```python
from build123d import *

# Parameters (mm, degrees)
SKETCH2_W               = 152.4
SKETCH2_H               = 44.45
BASE_FLANGE1_DEPTH      = 6.07314
CUT_EXTRUDE1_DEPTH      = 159.86612455
CUT_EXTRUDE1_DEPTH_BACK = 159.86612455


# Sheet-metal steps are written as plain solids
with BuildPart() as part:
    # Sketch2 → Base-Flange1 (new body)
    with BuildSketch(Plane(origin=(0, 0, 0), x_dir=(1, 0, 0), z_dir=(0, 1, 0))):
        with Locations((76.2, 22.225)):
            Rectangle(SKETCH2_W, SKETCH2_H)
    extrude(amount=-BASE_FLANGE1_DEPTH)

    # Sketch7 → Cut-Extrude1 (cut, two sides: drawn at the far end of the back side and taken through both)
    with BuildSketch(Plane.XZ.offset(6.07314).offset(-CUT_EXTRUDE1_DEPTH_BACK)):
        with BuildLine():
            Line((121.046875, -27.42184), (126.603125, -27.42184))
            ThreePointArc((126.603125, -27.42184), (132.953125, -21.07184), (126.603125, -14.72184))
            Line((126.603125, -14.72184), (121.046875, -14.72184))
            ThreePointArc((121.046875, -14.72184), (114.696875, -21.07184), (121.046875, -27.42184))
        make_face()
        with BuildLine():
            Line((31.353125, -14.72184), (25.796875, -14.72184))
            ThreePointArc((25.796875, -14.72184), (19.446875, -21.07184), (25.796875, -27.42184))
            Line((25.796875, -27.42184), (31.353125, -27.42184))
            ThreePointArc((31.353125, -27.42184), (37.703125, -21.07184), (31.353125, -14.72184))
        make_face()
    extrude(amount=CUT_EXTRUDE1_DEPTH + CUT_EXTRUDE1_DEPTH_BACK, mode=Mode.SUBTRACT)


solid = part.part
```
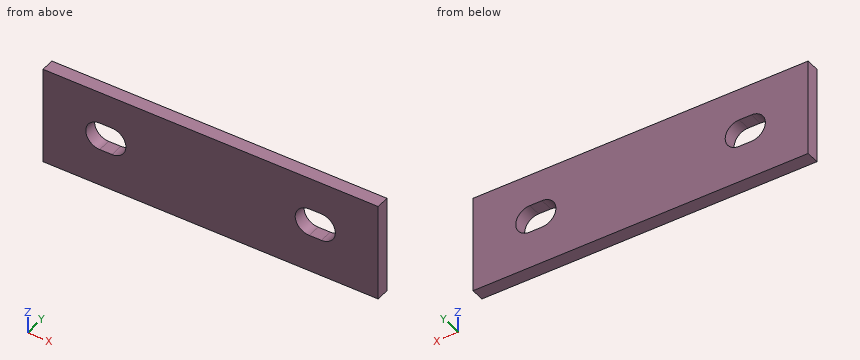
The model under review builds one solid part; all positions refer to its coordinate system, in mm. Round coordinates to 2 decimals unless told otherwise and drop trailing zeros. Write each loop counter-clockwise with the first axis right and the second up, starting at its lowest first coordinate (ties: lowest second). Pieces come first, ordered by that corner, then holes. Notation, with made-up numbers: M -33.75,-39 L -12.75,-39 A22 cw -12.75,-32 Z; hole C -2,72.5 d3. An arc over 180 degrees is marked long. Use CSV: the item, a comma, the result in double quotes. Start each with the question number.
(1) We need section B-B, the plane y = -2.75. State the section outline as (x, z) points.
(2) For line 1 along Z through (x, y) = (28, -5); line 2 along X through (y, z) = (-3.25, -24); line 3 along X through (y, z) = (-4.75, -23.5), list the stretches that pass through material, from the lowest coordinate up.
(3) We need section A-A, the plane x = 117.5. State the section outline as (y, z) points, then the cut area to 3 significant figures.
(4) We need section C-C, the plane z = -24. State the section outline as (x, y) points.
Findings:
1,outline,"M 0,-44.45 L 152.4,-44.45 L 152.4,0 L 0,0 Z; hole M 25.8,-27.42 L 31.35,-27.42 A6.35 ccw 31.35,-14.72 L 25.8,-14.72 A6.35 ccw Z; hole M 121.05,-27.42 L 126.6,-27.42 A6.35 ccw 126.6,-14.72 L 121.05,-14.72 A6.35 ccw Z"
2,line 1,"-44.45 to -27.42, -14.72 to 0"
2,line 2,"0 to 20.16, 36.99 to 115.41, 132.24 to 152.4"
2,line 3,"0 to 19.93, 37.22 to 115.18, 132.47 to 152.4"
3,outline,"M -6.07,-44.45 L 0,-44.45 L 0,-26.34 L -6.07,-26.34 Z; M -6.07,-15.8 L 0,-15.8 L 0,0 L -6.07,0 Z"
3,area,"206 mm^2"
4,outline,"M 0,-6.07 L 20.16,-6.07 L 20.16,0 L 0,0 Z; M 36.99,-6.07 L 115.41,-6.07 L 115.41,0 L 36.99,0 Z; M 132.24,-6.07 L 152.4,-6.07 L 152.4,0 L 132.24,0 Z"
